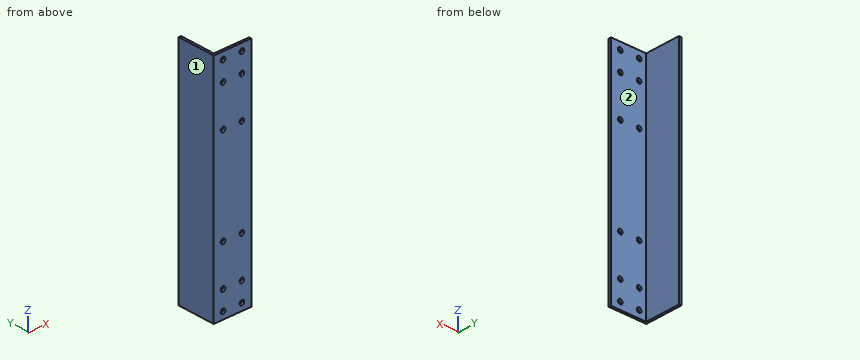
from build123d import *

# Parameters (mm, degrees)
BOSS_EXTRUDE1_DEPTH = 304.8
SKETCH2_R           = 3.175
CUT_EXTRUDE1_DEPTH  = 314.152231351


with BuildPart() as part:
    # Sketch1 → Boss-Extrude1 (new body)
    with BuildSketch(Plane.XY):
        Polygon((0, 0), (50.8, 0), (50.8, 3.175), (3.175, 3.175), (3.175, 50.8), (0, 50.8), align=None)
    extrude(amount=BOSS_EXTRUDE1_DEPTH)

    # Sketch2 → Cut-Extrude1 (cut, through all)
    with BuildSketch(Plane.XZ):
        with Locations(Location((12.7, 9.525, 0), (0, 0, 270))):
            Circle(SKETCH2_R)
        with Locations(Location((12.7, 34.925, 0), (0, 0, 270))):
            Circle(SKETCH2_R)
        with Locations(Location((38.1, 34.925, 0), (0, 0, 270))):
            Circle(SKETCH2_R)
        with Locations(Location((38.1, 9.525, 0), (0, 0, 270))):
            Circle(SKETCH2_R)
        with Locations(Location((12.7, 215.9, 0), (0, 0, 270))):
            Circle(SKETCH2_R)
        with Locations(Location((38.1, 215.9, 0), (0, 0, 270))):
            Circle(SKETCH2_R)
        with Locations(Location((38.1, 88.9, 0), (0, 0, 270))):
            Circle(SKETCH2_R)
        with Locations(Location((12.7, 88.9, 0), (0, 0, 270))):
            Circle(SKETCH2_R)
        with Locations(Location((12.7, 295.275, 0), (0, 0, 270))):
            Circle(SKETCH2_R)
        with Locations(Location((12.7, 269.875, 0), (0, 0, 270))):
            Circle(SKETCH2_R)
        with Locations(Location((38.1, 269.875, 0), (0, 0, 270))):
            Circle(SKETCH2_R)
        with Locations(Location((38.1, 295.275, 0), (0, 0, 270))):
            Circle(SKETCH2_R)
    extrude(amount=-CUT_EXTRUDE1_DEPTH, mode=Mode.SUBTRACT)


solid = part.part
Could you check a few things on this model? Use its own coordinates, in mm. Face numbers are marked on the shaded views. A direction names the side the tool comes from. Give positions to 0.01 mm unless a question says otherwise; leave off trailing zeros. Order: outer loops, then holes, each group sorted by start corner. A loop starts at its lowest first (then second) coordinate and runs counter-clockwise, first axis right, second up. Notation, with made-up numbers: (21, 43.25) -> (54, 43.25) arc R23 cw to (54, 80.25) -> close; hole circle Ø9 at (-19.75, -21). An arc over 180 degrees is marked (long way). Answer in a Markdown table with one row per item. Add a question column.
Item 1: I'm going to push flat-ended pins straight in: P1, Ø1.5, axis at y = 26, z = 125, coming from the +X side (3 decimals); P2, Ø14.5, axis at x = 23.5, z = 222, coming from the +Y side (3 decimals); P3, Ø4, axis at x = 38.1, z = 34.925, coming from the -Y side. Where does each tip first touch, or does it pass through?
Item 2: For the marked faces 1 and 2, which set-ups out of +Z, -Z, +X, -X, +Y, -Y let a thin tool reach every point of the face, with its end or its side?
Item 3: Please list where these lines run through material, in increasing order: probe 1 along X at (y, z) = (2, 88); probe 2 along Y at (x, z) = (18, 197) (3 decimals).
Item 4: Imagine slicing it at C-C (y = 11). List the corners of the cut face in (x, z) for me (3 decimals), and give its area (3 significant figures).
Item 5: Imagine slicing it at A-A (x = 38.1). List the corners of the cut face in (y, z) for me (3 decimals), and give its area (3 significant figures).
Item 6: Imagine slicing it at B-B (z = 215.9). List the corners of the cut face in (x, y) for me (3 decimals), and give its area (3 significant figures).
Result:
| question | item | result |
|---|---|---|
| 1 | P1 | x = 3.175 |
| 1 | P2 | y = 3.175 |
| 1 | P3 | through |
| 2 | face 1 | +Z, -Z, -X, +Y, -Y |
| 2 | face 2 | +Z, -Z, +X, +Y |
| 3 | probe 1 | 0 to 9.66, 15.74 to 35.06, 41.14 to 50.8 |
| 3 | probe 2 | 0 to 3.175 |
| 4 | outline | (0, 0) -> (3.175, 0) -> (3.175, 304.8) -> (0, 304.8) -> close |
| 4 | area | 968 mm2 |
| 5 | outline | (0, 0) -> (3.175, 0) -> (3.175, 6.35) -> (0, 6.35) -> close; (0, 12.7) -> (3.175, 12.7) -> (3.175, 31.75) -> (0, 31.75) -> close; (0, 38.1) -> (3.175, 38.1) -> (3.175, 85.725) -> (0, 85.725) -> close; (0, 92.075) -> (3.175, 92.075) -> (3.175, 212.725) -> (0, 212.725) -> close; (0, 219.075) -> (3.175, 219.075) -> (3.175, 266.7) -> (0, 266.7) -> close; (0, 273.05) -> (3.175, 273.05) -> (3.175, 292.1) -> (0, 292.1) -> close; (0, 298.45) -> (3.175, 298.45) -> (3.175, 304.8) -> (0, 304.8) -> close |
| 5 | area | 847 mm2 |
| 6 | outline | (0, 0) -> (9.525, 0) -> (9.525, 3.175) -> (3.175, 3.175) -> (3.175, 50.8) -> (0, 50.8) -> close; (15.875, 0) -> (34.925, 0) -> (34.925, 3.175) -> (15.875, 3.175) -> close; (41.275, 0) -> (50.8, 0) -> (50.8, 3.175) -> (41.275, 3.175) -> close |
| 6 | area | 272 mm2 |
